Geometry check sheet. Reference: the model listing, model coordinates, mm. A direction names the side the tool comes from. Round coordinates to 2 decimals unless told otherwise and drop trailing zeros. Loops run counter-clockwise (first coordinate to the right, second up) from the corner with the lowest first, then second, coordinate; pieces in that order, holes last. Notation, with made-up numbers: (44.5, -17.75) -> (96.5, -17.75) arc R23 ccw to (96.5, 5.25) -> close; hole circle Ø6 at (43, -27). An arc over 180 degrees is marked (long way). Use a Markdown table: item, result. Add a question column.
Q1. Gauge pin test, flat ends, axial feed: P1, Ø1, axis at x = -5.5, y = -5, coming from the -Z side; P2, Ø12, axis at x = 6.5, z = 41.5, coming from the +Y side; P3, Ø6, axis at x = 4.5, z = 29, coming from the +Y side; P4, Ø3, axis at y = 12.5, z = 12, coming from the +X side. Record the tip position at first contact, or that the pin passes through.
Q2. Sectioned sample at A-A, the plane y = 0. Enter the section's corners in (x, z), then the cut area to 3 significant figures.
Q3. Sectioned sample at C-C, the plane z = 37.5. Enter the section's corners in (x, y).
Q4. Release check for a two-part mould opening along X. For faces 1 (the face through (-13.887, -10.648, 7.479)), 2 (the face through (5, 3, 15)), 3 (the face through (-0.37, -1.66, 31.1)) record: released by +X, released by -X, zero draft, split by the parting line, or undercut.
Q5. Set-up check for faces 4 (the face through (-0.54, -2.44, 38.71)), 5 (the face through (5, 0, 0)): record each of +Z, -Z, +X, -X, +Y, -Y from which the full face is reachable in a straight line by a thin tool's end or side.
Q6. Material ranges on L1, parallel to Y at x = 0, z = 43; L2, parallel to Z at x = 5, y = 5; L3, parallel to Y at x = 0, z = 13, recorded low to high.
```python
from build123d import *

# Parameters (mm, degrees)
F0_R     = 17.5
F0_R_2   = 2.5
F1_DEPTH = 15
F2_R     = 6
F0_R_3   = 1.7
F3_DEPTH = 60
F4_R     = 3


with BuildPart() as f1:
    # F0 (on Top) → F1 (new body)
    with BuildSketch(Plane.XY):
        Circle(F0_R)
        Circle(F0_R_2, mode=Mode.SUBTRACT)
    extrude(amount=F1_DEPTH)

    # F2
    f2_edges = [f1.edges().sort_by_distance(p)[0] for p in [
        (-17.5, 0, 15),
        (-17.5, 0, 0),
    ]]
    fillet(f2_edges, radius=F2_R)

    # F0 (on Top) → F3 (join)
    with BuildSketch(Plane.XY):
        Circle(F0_R_2)
        Circle(F0_R_3, mode=Mode.SUBTRACT)
    extrude(amount=F3_DEPTH)

    # F4
    f4_edges = [f1.edges().sort_by_distance(p)[0] for p in [
        (-1.7, 0, 0),
        (-2.5, 0, 15),
    ]]
    fillet(f4_edges, radius=F4_R)


solid = f1.part
```
Values:
| question | item | result |
|---|---|---|
| 1 | P1 | z = 0 |
| 1 | P2 | y = 2.45 |
| 1 | P3 | y = 2 |
| 1 | P4 | x = 12.87 |
| 2 | outline | (-17.5, 6) arc R6 ccw to (-11.5, 0) -> (-4.7, 0) arc R3 ccw to (-1.7, 3) -> (-1.7, 60) -> (-2.5, 60) -> (-2.5, 18) arc R3 cw to (-5.5, 15) -> (-11.5, 15) arc R6 ccw to (-17.5, 9) -> close; (1.7, 3) arc R3 ccw to (4.7, 0) -> (11.5, 0) arc R6 ccw to (17.5, 6) -> (17.5, 9) arc R6 ccw to (11.5, 15) -> (5.5, 15) arc R3 cw to (2.5, 18) -> (2.5, 60) -> (1.7, 60) -> close |
| 2 | area | 515 mm^2 |
| 3 | outline | circle Ø5 at (0, 0); hole circle Ø3.4 at (0, 0) |
| 4 | face 1 | split by the parting line |
| 4 | face 2 | zero draft |
| 4 | face 3 | undercut |
| 5 | face 4 | +Z |
| 5 | face 5 | -Z, +X, -X, +Y, -Y |
| 6 | L1 | -2.5 to -1.7, 1.7 to 2.5 |
| 6 | L2 | 0 to 15 |
| 6 | L3 | -15.97 to -1.7, 1.7 to 15.97 |
